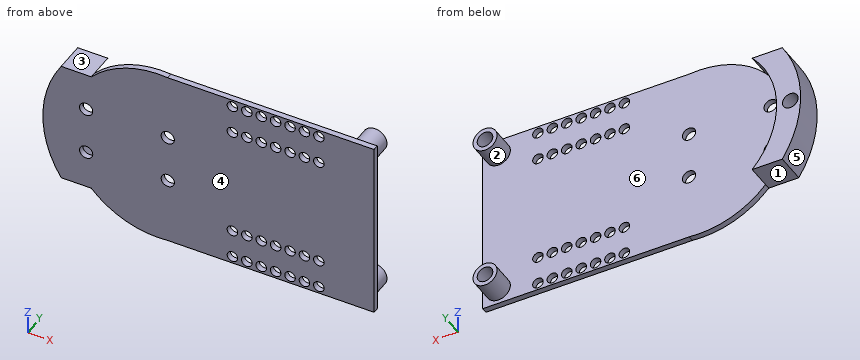
Autodesk Inventor part; units mm, degrees
ref_plane "YZ Plane" through (0, 0, 0) normal (1, 0, 0) x (0, 1, 0)
ref_plane "XZ Plane" through (0, 0, 0) normal (0, 1, 0) x (-1, 0, 0)
ref_plane "XY Plane" through (0, 0, 0) normal (0, 0, 1) x (1, 0, 0)
sketch "Sketch1" plane through (0, 0, 0) normal (0, 1, 0) x (-1, 0, 0)
  line L0 (0, 0) -> (86, 0)
  line L1 (0, 0) -> (0, -76)
  line L2 (86, -76) -> (0, -76)
  arc A0 (86, -76) -> (86, 0) centre (89.8131, -38) ccw
  line L3 (86, -76) -> (86, -86)
  line L4 (86, 0) -> (86, 10)
  arc A1 (130.3413, -64) -> (130.3413, -12) centre (89.8131, -38) ccw
  line L5 (86, 0) -> (86, -12)
  line L6 (86, -76) -> (86, -64)
  line L7 (117.787, -12) -> (130.3413, -12)
  line L8 (117.787, -64) -> (130.3413, -64)
  line L9 (117.787, -12) -> (130.3413, -12)
  line L10 (117.787, -64) -> (130.3413, -64)
  line L11 (130.3413, -12) -> (117.787, -12)
  line L12 (130.3413, -64) -> (117.787, -64)
  arc A2 (117.787, -64) -> (117.787, -12) centre (89.8131, -38) ccw
  arc A3 (130.3413, -64) -> (130.3413, -12) centre (89.8131, -38) ccw
  dimension "d1" = 86
  dimension "d2" = 76
  dimension "d3" = 10
  dimension "d4" = 10
  dimension "d6" = 12
  dimension "d7" = 12
extrude "Extrusion1" add sketch "Sketch1" along normal blind 2.4
sketch "Sketch2" plane through (0, 2.4, 0) normal (0, 1, 0) x (1, 0, 0)
  circle A0 centre (-6.5, 6.5) radius 5
  circle A1 centre (-6.5, 69.5) radius 5
  line L0 (-86, 0) -> (0, 0)
  line L1 (0, 0) -> (0, 76)
  arc A2 (-117.787, 64) -> (-117.787, 12) centre (-89.7207, 38) ccw
  line L2 (-130.3413, 12) -> (-117.787, 12)
  line L3 (-130.3413, 12) -> (-117.787, 12)
  line L4 (-117.787, 64) -> (-130.3413, 64)
  line L5 (-130.3413, 64) -> (-117.787, 64)
  arc A3 (-130.3413, 64) -> (-130.3413, 12) centre (-89.8131, 38) ccw
  dimension "d10" = 10
  dimension "d11" = 10
  dimension "d12" = 63
  dimension "d13" = 6.5
  dimension "d14" = 6.5
  dimension "d15" = 6.5
extrude "Extrusion2" add sketch "Sketch2" along normal blind 10
sketch "Sketch4" plane through (-6.5, 12.4, -6.5) normal (0, 1, 0) x (1, 0, 0)
  circle A0 centre (0, 0) radius 3.25
  circle A1 centre (0, 63) radius 5
  circle A2 centre (0, 63) radius 3.25
  line L0 (0, 0) -> (0, 63)
  line L1 (6.5, -6.5) -> (6.5, 69.5)
  line L2 (0, 31.5) -> (-127.167, 31.5)
  circle A3 centre (-127.167, 31.5) radius 3.25
  dimension "d20" = 6.5
  dimension "d21" = 6.5
  dimension "d22" = 127.167
  dimension "d23" = 6.5
  dimension "d70" = 63
hole "Hole1" at (-133.667, 12.4, -38) at (-6.5, 12.4, -69.5) at (-6.5, 12.4, -6.5) direction (0, -1, 0) diameter 6.5 depth 9
sketch "Sketch5" plane through (0, 2.4, 0) normal (0, 1, 0) x (1, 0, 0)
  line L0 (-86, 0) -> (0, 0)
  line L1 (-55.3616, 0) -> (-55.3616, 76)
  line L2 (0, 76) -> (-86, 76)
  line L3 (-55.3616, 38) -> (-127.9792, 38)
  arc A0 (-117.787, 64) -> (-117.787, 12) centre (-89.7207, 38) ccw
  arc A1 (-117.787, 64) -> (-117.787, 12) centre (-89.7207, 38) ccw
  arc A2 (-117.787, 12) -> (-86, 0) centre (-89.8131, 38) ccw
  line L4 (-86, 0) -> (0, 0)
  line L5 (0, 0) -> (0, 76)
  line L6 (0, 76) -> (-86, 76)
  arc A3 (-86, 76) -> (-117.787, 64) centre (-89.8131, 38) ccw
  circle A4 centre (-6.5, 69.5) radius 5
  circle A5 centre (-6.5, 6.5) radius 5
  circle A6 centre (-119.9244, 28) radius 2.75
  line L7 (-119.9244, 28) -> (-119.9244, 38)
  circle A7 centre (-119.9244, 48) radius 2.75
  circle A8 centre (-85.9244, 28) radius 2.75
  circle A9 centre (-85.9244, 48) radius 2.75
  dimension "d36" = 5.5
  dimension "d38" = 5.5
  dimension "d39" = 10
  dimension "d40" = 10
  dimension "d41" = 5.5
  dimension "d42" = 5.5
  dimension "d43" = 34
  dimension "d44" = 34
hole "Hole2" at (-119.9244, 2.4, -28) at (-119.9244, 2.4, -48) at (-85.9244, 2.4, -48) at (-85.9244, 2.4, -28) direction (0, -1, 0) diameter 5.5 end through all
sketch "Sketch6" plane through (0, 2.4, 0) normal (0, 1, 0) x (1, 0, 0)
  line L0 (-16.1203, 0) -> (-16.1203, 27)
  circle A0 centre (-23, 61) radius 2.2
  line L1 (0, 0) -> (0, 76)
  line L2 (0, 76) -> (-86, 76)
  circle A1 centre (-35, 61) radius 2.2
  circle A2 centre (-47, 61) radius 2.2
  circle A3 centre (-59, 61) radius 2.2
  line L3 (0, 0) -> (0, 76)
  line L4 (0, 38) -> (-47, 38)
  circle A4 centre (-23, 15) radius 2.2
  circle A5 centre (-35, 15) radius 2.2
  circle A6 centre (-47, 15) radius 2.2
  circle A7 centre (-59, 15) radius 2.2
  line L5 (-47, 38) -> (-86, 38)
  line L6 (-35, 61) -> (-35, 73)
  circle A8 centre (-35, 73) radius 2.2
  circle A9 centre (-47, 73) radius 2.2
  circle A10 centre (-35, 3) radius 2.2
  circle A11 centre (-47, 3) radius 2.2
  circle A12 centre (-53, 61) radius 2.2
  circle A13 centre (-41, 61) radius 2.2
  circle A14 centre (-29, 61) radius 2.2
  line L7 (-47, 61) -> (-47, 73)
  line L8 (-47, 67) -> (-37.2, 67)
  circle A15 centre (-23, 73) radius 2.2
  circle A16 centre (-35, 73) radius 2.2
  circle A17 centre (-47, 73) radius 2.2
  circle A18 centre (-59, 73) radius 2.2
  line L9 (-35, 73) -> (-35, 61)
  circle A19 centre (-53, 73) radius 2.2
  circle A20 centre (-41, 73) radius 2.2
  circle A21 centre (-29, 73) radius 2.2
  circle A22 centre (-23, 15) radius 2.2
  circle A23 centre (-35, 15) radius 2.2
  circle A24 centre (-47, 15) radius 2.2
  circle A25 centre (-59, 15) radius 2.2
  circle A26 centre (-35, 3) radius 2.2
  circle A27 centre (-53, 15) radius 2.2
  circle A28 centre (-41, 15) radius 2.2
  circle A29 centre (-29, 15) radius 2.2
  circle A30 centre (-59, 3) radius 2.2
  circle A31 centre (-53, 3) radius 2.2
  circle A32 centre (-47, 3) radius 2.2
  circle A33 centre (-41, 3) radius 2.2
  circle A34 centre (-29, 3) radius 2.2
  circle A35 centre (-23, 3) radius 2.2
  dimension "d52" = 27
  dimension "d54" = 4.4
  dimension "d57" = 4.4
  dimension "d59" = 4.4
  dimension "d61" = 4.4
  dimension "d71" = 23
  dimension "d73" = 23
  dimension "d74" = 23
  dimension "d75" = 23
  dimension "d76" = 12
  dimension "d77" = 4.4
  dimension "d78" = 4.4
  dimension "d79" = 4.4
  dimension "d80" = 6
  dimension "d81" = 4.4
  dimension "d82" = 6
  dimension "d83" = 4.4
  dimension "d84" = 6
hole "Hole3" at (-59, 2.4, -15) at (-47, 2.4, -15) at (-35, 2.4, -15) at (-23, 2.4, -15) at (-23, 2.4, -61) at (-35, 2.4, -61) at (-47, 2.4, -61) at (-59, 2.4, -61) at (-47, 2.4, -3) at (-35, 2.4, -3) at (-35, 2.4, -73) at (-47, 2.4, -73) at (-59, 2.4, -3) at (-53, 2.4, -3) at (-53, 2.4, -15) at (-41, 2.4, -15) at (-41, 2.4, -3) at (-29, 2.4, -3) at (-23, 2.4, -3) at (-29, 2.4, -15) at (-59, 2.4, -73) at (-53, 2.4, -73) at (-53, 2.4, -61) at (-41, 2.4, -61) at (-41, 2.4, -73) at (-29, 2.4, -73) at (-29, 2.4, -61) at (-23, 2.4, -73) direction (0, -1, 0) diameter 4.4 end through all
properties part number "baseChassis322016"
Build history of the part. All positions in model axes, mm. Face numbers are marked on the shaded views. A direction names the side the tool comes from. Round coordinates to 2 decimals unless told otherwise and drop trailing zeros. Write each loop counter-clockwise with the first axis right and the second up, starting at its lowest first coordinate (ties: lowest second). Pieces come first, ordered by that corner, then holes. Notation, with made-up numbers: M 8.25,-38 L 48.25,-38 A31 cw 48.25,-12 Z; hole C 54.25,51.5 d2. An arc over 180 degrees is marked long. Answer in a Markdown table with one row per item.
1. Probe L1, parallel to Z at x = -47, y = 0.8; L2, parallel to X at y = 1.9, z = -48; L3, parallel to Z at x = -6.5, y = 9.25. List the from-to ranges inside material, lowest first. Write a range as [from, to].
Geometry check:
| item | result |
|---|---|
| L1 | [-76, -75.2], [-70.8, -63.2], [-58.8, -17.2], [-12.8, -5.2], [-0.8, 0] |
| L2 | [-136.91, -122.67], [-117.17, -88.67], [-83.17, 0] |
| L3 | [-74.5, -72.75], [-66.25, -64.5], [-11.5, -9.75], [-3.25, -1.5] |
2. Saw through at C-C (z = -48). List the corners of the cut face in (x, y).
Geometry check:
| item | result |
|---|---|
| outline | M -136.91,0 L -122.67,0 L -122.67,2.4 L -126.65,2.4 L -126.65,12.4 L -136.91,12.4 Z; M -117.17,0 L -88.67,0 L -88.67,2.4 L -117.17,2.4 Z; M -83.17,0 L 0,0 L 0,2.4 L -83.17,2.4 Z |
3. Saw through at B-B (y = 7.5). List the corners of the cut face in (x, z), and give its area (3 significant figures).
Geometry check:
| item | result |
|---|---|
| outline | M -130.34,-64 L -117.79,-64 A38.26 cw -117.79,-12 L -130.34,-12 A48.15 ccw Z; C -6.5,-69.5 d10; C -6.5,-6.5 d10; hole C -133.67,-38 d6.5; hole C -6.5,-69.5 d6.5; hole C -6.5,-6.5 d6.5 |
| area | 615 mm2 |
4. Saw through at D-D (z = -38). List the corners of the cut face in (x, y), and give its area (3 significant figures).
Geometry check:
| item | result |
|---|---|
| outline | M -137.96,0 L 0,0 L 0,2.4 L -127.98,2.4 L -127.98,12.4 L -130.42,12.4 L -130.42,3.4 L -136.92,3.4 L -136.92,12.4 L -137.96,12.4 Z |
| area | 372 mm2 |
5. Mould opens along Z. For the marked faces 1, 2, 3 and 4 say: +Z half, -Z half, draft (parallel to the pull), parting line (faces both ways), or undercut.
Geometry check:
| item | result |
|---|---|
| face 1 | -Z half |
| face 2 | undercut |
| face 3 | +Z half |
| face 4 | draft |
6. Which spindle directions (+Z, -Z, +X, -X, +Y, -Y) get a long thin tool onto all of the face, cutting with end or side? Do the marked faces 5 and 6. Say none if no direction does.
Geometry check:
| item | result |
|---|---|
| face 5 | -X, +Y, -Y |
| face 6 | +Y |
7. Flat gauge pins, fed straight in: P1, Ø3, axis at x = -132.5, z = -38.5, coming from the +Y side; P2, Ø1.5, axis at y = 7.5, z = -27, coming from the +X side; P3, Ø10, axis at x = -31.5, z = -21, coming from the +Y side. Where does each tip first touch, or does it go through?
Geometry check:
| item | result |
|---|---|
| P1 | y = 3.4 |
| P2 | x = -126.13 |
| P3 | y = 2.4 |
8. Saw through at A-A (x = -35). List the corners of the cut face in (y, z), and give its area (3 significant figures).
Geometry check:
| item | result |
|---|---|
| outline | M 0,-76 L 2.4,-76 L 2.4,-75.2 L 0,-75.2 Z; M 0,-70.8 L 2.4,-70.8 L 2.4,-63.2 L 0,-63.2 Z; M 0,-58.8 L 2.4,-58.8 L 2.4,-17.2 L 0,-17.2 Z; M 0,-12.8 L 2.4,-12.8 L 2.4,-5.2 L 0,-5.2 Z; M 0,-0.8 L 2.4,-0.8 L 2.4,0 L 0,0 Z |
| area | 140 mm2 |
